Here's how the part is built. I have some questions about the finished solid (model axes, mm). A direction names the side the tool comes from. Give positions to 0.01 mm unless a question says otherwise; leave off trailing zeros. Order: outer loops, then holes, each group sorted by start corner. A loop starts at its lowest first (then second) coordinate and runs counter-clockwise, first axis right, second up. Notation, with made-up numbers: (79.25, -4.75) - (125.25, -4.75) arc R36 ccw to (125.25, 29.25) - close; hole circle Ø3 at (50.5, -21). An arc over 180 degrees is marked (long way). One line per question, with ' | ' between items.
from build123d import *

# Parameters (mm, degrees)
SKETCH_2_R               = 1.5
CUT_EXTRUDE_1_DEPTH      = 10
CUT_EXTRUDE_2_DEPTH      = 87.835131139
CUT_EXTRUDE_2_DEPTH_BACK = 87.835131139
SKETCH_3_W               = 1
SKETCH_3_H               = 14


with BuildPart() as part:
    # 草图1 → 旋转1 (revolve)
    with BuildSketch(Plane(origin=(0, 0, 0), x_dir=(0, 0, -1), z_dir=(1, 0, 0)), mode=Mode.PRIVATE) as revolve_1_sk:
        Polygon((0, 0), (0, 3), (14, 3), (14, 6), (19, 6), (19, 18.5), (49.5, 18.5), (49.5, 18), (82.8, 18), (82.8, 0), align=None)
    revolve(revolve_1_sk.sketch.rotate(Axis((0, 0, 0), (0, 0, -1)), 90), axis=Axis((0, 0, 0), (0, 0, -1)))

    # 草图2 → 切除-拉伸1 (cut)
    with BuildSketch(Plane.XY.offset(-19)):
        with Locations((0, 15.5)):
            Circle(SKETCH_2_R)
        with Locations((13.423393759, 7.75)):
            Circle(SKETCH_2_R)
        with Locations((13.423393759, -7.75)):
            Circle(SKETCH_2_R)
        with Locations((0, -15.5)):
            Circle(SKETCH_2_R)
        with Locations((-13.423393759, -7.75)):
            Circle(SKETCH_2_R)
        with Locations((-13.423393759, 7.75)):
            Circle(SKETCH_2_R)
    extrude(amount=-CUT_EXTRUDE_1_DEPTH, mode=Mode.SUBTRACT)

    # 草图3 → 切除-拉伸2 (cut, two sides: drawn at the far end of the back side and taken through both)
    with BuildSketch(Plane(origin=(0, 0, 0), x_dir=(1, 0, 0), z_dir=(0, 1, 0)).offset(-CUT_EXTRUDE_2_DEPTH_BACK)):
        with Locations((3, 7)):
            Rectangle(SKETCH_3_W, SKETCH_3_H)
    extrude(amount=CUT_EXTRUDE_2_DEPTH + CUT_EXTRUDE_2_DEPTH_BACK, mode=Mode.SUBTRACT)


solid = part.part
1) I'm going to push flat-ended pins straight in: P1, Ø8, axis at x = 10, z = -53.5, coming from the -Y side; P2, Ø6, axis at x = 2, y = 10, coming from the +Z side; P3, Ø5, axis at y = -11.5, z = -34, coming from the -X side. Where does each tip first touch, or does it pass through?
Model answer:
P1: stops at y = -16.97 | P2: stops at z = -19 | P3: stops at x = -16.16
2) I want a section at A-A (x = 0). List the corners of the cut face in (y, z) for me, plus the area to 3 significant figures.
Model answer:
outline: (-18.5, -49.5) - (-18, -49.5) - (-18, -82.8) - (18, -82.8) - (18, -49.5) - (18.5, -49.5) - (18.5, -19) - (17, -19) - (17, -29) - (14, -29) - (14, -19) - (6, -19) - (6, -14) - (3, -14) - (3, 0) - (-3, 0) - (-3, -14) - (-6, -14) - (-6, -19) - (-14, -19) - (-14, -29) - (-17, -29) - (-17, -19) - (-18.5, -19) - close | area: 2,410 mm2
3) I want a section at B-B (y = 4.5). List the corners of the cut face in (x, z) for me, plus the area to 3 significant figures.
Model answer:
outline: (-17.94, -49.5) - (-17.43, -49.5) - (-17.43, -82.8) - (17.43, -82.8) - (17.43, -49.5) - (17.94, -49.5) - (17.94, -19) - (3.97, -19) - (3.97, -14) - (-3.97, -14) - (-3.97, -19) - (-17.94, -19) - close | area: 2,300 mm2
4) I want a section at C-C (z = -63). List the corners of the cut face in (x, y) for me, plus the area to 3 significant figures.
Model answer:
outline: circle Ø36 at (0, 0) | area: 1,020 mm2
5) On a 3-axis mill with a long thin cutter (end or side, diameter ignored), from which of +Z, -Z, +X, -X, +Y, -Y can I reach the whole of each face in a straight line? I mean faces 4 (the face through (-13.267, -12.165, -66.383)), 5 (the face through (8.54, 16.41, -34.46)), 6 (the face through (0, 0, -82.8)), 7 (the face through (-13.749, 6.286, -23.93)), 8 (the face through (2.5, 0, -7)). Say none if no direction works.
Model answer:
face 4: -Z | face 5: +Z, -Z | face 6: -Z, +X, -X, +Y, -Y | face 7: +Z | face 8: +Z, +X, +Y, -Y
6) I want a section at D-D (y = 0). List the corners of the cut face in (x, z) for me, plus the area to 3 significant figures.
Model answer:
outline: (-18.5, -49.5) - (-18, -49.5) - (-18, -82.8) - (18, -82.8) - (18, -49.5) - (18.5, -49.5) - (18.5, -19) - (6, -19) - (6, -14) - (2.5, -14) - (2.5, 0) - (-3, 0) - (-3, -14) - (-6, -14) - (-6, -19) - (-18.5, -19) - close | area: 2,460 mm2
7) Please list where these lines run through material, in increasing order: L1, parallel to Y at x = 0, z = -25; L2, parallel to Z at x = -7.5, y = 12; L3, parallel to X at y = 8, z = -22.
Model answer:
L1: y = -18.5 to -17, -14 to 14, 17 to 18.5 | L2: z = -82.8 to -19 | L3: x = -16.68 to -14.9, -11.94 to 11.94, 14.9 to 16.68
8) Thinking about a two-plate mould opening in Y: for faces 1 (the face through (-3, 0, -7)), 2 (the face through (-13.749, -9.214, -23.93)), 3 (the face through (4.4, -4.4, -19)), which applies, +Y half, -Y half, draft (parallel to the pull), parting line (faces both ways), or undercut?
Model answer:
face 1: parting line | face 2: undercut | face 3: draft
